Input: part model. Units: mm. Frame: model coordinates. A direction names the side the tool comes from. Coordinates: 2 decimals unless noted, no trailing zeros. Order: outer loops, then holes, each group sorted by start corner. A loop starts at its lowest first (then second) coordinate and runs counter-clockwise, first axis right, second up. Notation, with made-up numbers: (67.25, 16) -> (98.25, 16) arc R17 cw to (98.25, 49) -> close; hole circle Ø4 at (72.25, 31). An arc over 180 degrees is marked (long way). Write each question's results on one line, items separated by ' | '.
```python
from build123d import *

# Parameters (mm, degrees)
SKETCH1_R           = 4
BOSS_EXTRUDE1_DEPTH = 6
CUT_EXTRUDE1_REACH  = 18.031
SKETCH4_R           = 4.99
SKETCH6_R           = 6
CUT_EXTRUDE3_DEPTH  = 1


with BuildPart() as part:
    # Sketch1 → Boss-Extrude1 (new body)
    with BuildSketch(Plane.XY):
        with BuildLine():
            Line((-2.438559793, 7.619279896), (5, 10))
            Line((5, 10), (11, 10))
            Line((11, 10), (11, -10))
            Line((11, -10), (5, -10))
            Line((5, -10), (-2.438559793, -7.619279896))
            ThreePointArc((-2.438559793, -7.619279896), (-8, 0), (-2.438559793, 7.619279896))
        make_face()
        Circle(SKETCH1_R, mode=Mode.SUBTRACT)
    extrude(amount=BOSS_EXTRUDE1_DEPTH)

    # Sketch4 → Cut-Extrude1 (cut, up to next)
    with BuildSketch(Plane.XY.offset(6), mode=Mode.PRIVATE) as cut_extrude1_sk1:
        Circle(SKETCH4_R)
    cut_extrude1_tool1 = extrude(cut_extrude1_sk1.sketch, amount=-CUT_EXTRUDE1_REACH, mode=Mode.PRIVATE) & part.part
    add(cut_extrude1_tool1.solids().sort_by_distance((0, 0, 6))[0], mode=Mode.SUBTRACT)

    # Sketch6 → Cut-Extrude3 (cut)
    with BuildSketch(Plane(origin=(0, 0, 0), x_dir=(-1, 0, 0), z_dir=(0, 0, -1))):
        Circle(SKETCH6_R)
    extrude(amount=-CUT_EXTRUDE3_DEPTH, mode=Mode.SUBTRACT)


solid = part.part
```
(1) Cut plane A-A, the plane y = 0. Return loops of the section in (x, z), plus the area to 3 significant figures.
Return value:
outline: (-8, 0) -> (-6, 0) -> (-6, 1) -> (-4.99, 1) -> (-4.99, 6) -> (-8, 6) -> close; (4.99, 1) -> (6, 1) -> (6, 0) -> (11, 0) -> (11, 6) -> (4.99, 6) -> close | area: 52.1 mm2
(2) Cut plane B-B, the plane z = 0.5. Return loops of the section in (x, y).
Return value:
outline: (-2.44, -7.62) -> (5, -10) -> (11, -10) -> (11, 10) -> (5, 10) -> (-2.44, 7.62) arc R8 ccw to start; hole circle Ø12 at (0, 0)
(3) Cut plane C-C, the plane x = 0. Return loops of the section in (y, z), plus the area to 3 significant figures.
Return value:
outline: (-8.4, 0) -> (-6, 0) -> (-6, 1) -> (-4.99, 1) -> (-4.99, 6) -> (-8.4, 6) -> close; (4.99, 1) -> (6, 1) -> (6, 0) -> (8.4, 0) -> (8.4, 6) -> (4.99, 6) -> close | area: 38.9 mm2
(4) Cut plane D-D, the plane z = 2.5. Return loops of the section in (x, y).
Return value:
outline: (-2.44, -7.62) -> (5, -10) -> (11, -10) -> (11, 10) -> (5, 10) -> (-2.44, 7.62) arc R8 ccw to start; hole circle Ø9.98 at (0, 0)
(5) Mould query, pull axis X, two halves, no side actions, for faces 1 (the face through (1.229, 8.793, 2.958)), 2 (the face through (11, 0, 3)), 3 (the face through (4, 4, 1)). Classes: +X half, -X half, draft (parallel to the pull), parting line (faces both ways), or undercut.
Return value:
face 1: -X half | face 2: +X half | face 3: undercut
(6) Pin query (flat end, axial travel): P1, Ø3.5, axis at x = 1, y = -2.5, coming from the -Z side; P2, Ø1, axis at x = -5, z = 1, coming from the -Y side; P3, Ø1, axis at y = -3, z = 5, coming from the -X side; P4, Ø1.5, axis at x = 2.5, z = 4.5, coming from the -Y side. Return the tip coordinate at first contact, or that it passes through.
Return value:
P1: through | P2: y = -6.61 | P3: x = -7.6 | P4: y = -9.44
(7) Reachability of faces 4 (the face through (5.994, 0.264, 0.493)), 5 (the face through (6, 0, 6)) from +Z, -Z, +X, -X, +Y, -Y: full face, straight path, thin tool, end or side. Return the list, or none.
Return value:
face 4: -Z | face 5: +Z, +X, -X, +Y, -Y
(8) Line query: line 1 along X through (y, z) = (-1.25, 4.55); line 2 along Y through (x, z) = (0, 0.5); line 3 along X through (y, z) = (1, 2.6). Output: solid intervals per line, ascending. Write a range as from..to.
Return value:
line 1: -7.9..-4.83, 4.83..11 | line 2: -8.4..-6, 6..8.4 | line 3: -7.94..-4.89, 4.89..11
